```python
from build123d import *

# Parameters (mm, degrees)
SKETCH1_W           = 155.575
SKETCH1_H           = 107.237500028
BOSS_EXTRUDE1_DEPTH = 36.5
SHELL2_T            = -3.175
FILLET1_R           = 2.54
CUT_EXTRUDE2_REACH  = 194.447
SKETCH7_R           = 1.2
SKETCH7_W           = 15
SKETCH7_H           = 15
SKETCH8_R           = 2.38125
CUT_EXTRUDE3_DEPTH  = 190.889155594


with BuildPart() as part:
    # Sketch1 → Boss-Extrude1 (new body)
    with BuildSketch(Plane(origin=(0, 0, 0), x_dir=(0, 0, -1), z_dir=(1, 0, 0))):
        with Locations((77.7875, 53.618750014)):
            Rectangle(SKETCH1_W, SKETCH1_H)
    extrude(amount=BOSS_EXTRUDE1_DEPTH)

    # Shell2
    shell2_openings = [part.faces().sort_by_distance(p)[0] for p in [
        (18.25, 53.618750014, 0),
    ]]
    offset(amount=SHELL2_T, openings=shell2_openings, kind=Kind.INTERSECTION)

    # Fillet1
    fillet1_edges = [part.edges().sort_by_distance(p)[0] for p in [
        (36.5, 107.237500028, -77.7875),
        (0, 107.237500028, -77.7875),
        (0, 0, -77.7875),
        (36.5, 0, -77.7875),
    ]]
    fillet(fillet1_edges, radius=FILLET1_R)

    # Sketch7 → Cut-Extrude2 (cut, up to next)
    with BuildSketch(Plane(origin=(0, 0, -155.575), x_dir=(-1, 0, 0), z_dir=(0, 0, -1)), mode=Mode.PRIVATE) as cut_extrude2_sk1:
        with Locations((-7.175, 30)):
            Circle(SKETCH7_R)
    cut_extrude2_tool1 = extrude(cut_extrude2_sk1.sketch, amount=-CUT_EXTRUDE2_REACH, mode=Mode.PRIVATE) & part.part
    # Sketch7 → Cut-Extrude2 (cut, up to next)
    with BuildSketch(Plane(origin=(0, 0, -155.575), x_dir=(-1, 0, 0), z_dir=(0, 0, -1)), mode=Mode.PRIVATE) as cut_extrude2_sk2:
        with Locations((-7.175, 5)):
            Circle(SKETCH7_R)
    cut_extrude2_tool2 = extrude(cut_extrude2_sk2.sketch, amount=-CUT_EXTRUDE2_REACH, mode=Mode.PRIVATE) & part.part
    # Sketch7 → Cut-Extrude2 (cut, up to next)
    with BuildSketch(Plane(origin=(0, 0, -155.575), x_dir=(-1, 0, 0), z_dir=(0, 0, -1)), mode=Mode.PRIVATE) as cut_extrude2_sk3:
        with Locations((-20.675, 27.5)):
            Rectangle(SKETCH7_W, SKETCH7_H)
    cut_extrude2_tool3 = extrude(cut_extrude2_sk3.sketch, amount=-CUT_EXTRUDE2_REACH, mode=Mode.PRIVATE) & part.part
    add(cut_extrude2_tool1.solids().sort_by_distance((7.175, 30, -155.575))[0], mode=Mode.SUBTRACT)
    add(cut_extrude2_tool2.solids().sort_by_distance((7.175, 5, -155.575))[0], mode=Mode.SUBTRACT)
    add(cut_extrude2_tool3.solids().sort_by_distance((20.675, 27.5, -155.575))[0], mode=Mode.SUBTRACT)

    # Sketch8 → Cut-Extrude3 (cut, through all)
    with BuildSketch(Plane.XY.offset(-152.4)):
        with Locations((7.175, 25.4)):
            Circle(SKETCH8_R)
    extrude(amount=-CUT_EXTRUDE3_DEPTH, mode=Mode.SUBTRACT)


solid = part.part
```
Geometry: final body of the model. Coordinates: model frame, mm. A direction names the side the tool comes from. Coordinates: 2 decimals unless noted, no trailing zeros. Order: outer loops, then holes, each group sorted by start corner. A loop starts at its lowest first (then second) coordinate and runs counter-clockwise, first axis right, second up.
Item 1: Section query A-A (x = 23.5). Output: boundary loops of the cut face in (y, z) (1 decimal).
Answer:
outline: (0, -155.6) - (20, -155.6) - (20, -152.4) - (3.2, -152.4) - (3.2, 0) - (0, 0) - close; (35, -155.6) - (107.2, -155.6) - (107.2, 0) - (104.1, 0) - (104.1, -152.4) - (35, -152.4) - close
Item 2: Draft query along X for faces 4 (the face through (28.175, 27, -154)), 5 (the face through (18, 107.238, -77)), 6 (the face through (36.5, 54, -77)), 7 (the face through (18, 53, -152.4)). Return one class per face: released by +X, released by -X, zero draft, split by the parting line, or undercut.
Answer:
face 4: undercut
face 5: zero draft
face 6: released by +X
face 7: undercut
Item 3: Material intervals for line 1 along Y through (x, z) = (28, -130) (1 decimal); line 2 along X through (y, z) = (51, -79.5) (3 decimals); line 3 along Z through (x, y) = (16.5, 12.5) (3 decimals), sorted ascending.
Answer:
line 1: y = 0 to 3.2, 104.1 to 107.2
line 2: x = 0 to 3.175, 33.325 to 36.5
line 3: z = -155.575 to -152.4
Item 4: Contact query for a flat-ended pin moving along its axis: P1, Ø4, axis at x = 8.5, y = 41, coming from the +Z side. Output: stop coordinate, or through.
Answer:
P1: stops at z = -152.4
Item 5: Section query D-D (y = 25.4). Output: boundary loops of the cut face in (x, z) (3 decimals).
Answer:
outline: (0, -155.575) - (4.794, -155.575) - (4.794, -152.4) - (3.175, -152.4) - (3.175, 0) - (0, 0) - close; (9.556, -155.575) - (13.175, -155.575) - (13.175, -152.4) - (9.556, -152.4) - close; (28.175, -155.575) - (36.5, -155.575) - (36.5, 0) - (33.325, 0) - (33.325, -152.4) - (28.175, -152.4) - close
Item 6: Section query B-B (z = -138). Output: boundary loops of the cut face in (x, y) (1 decimal).
Answer:
outline: (0, 2.5) arc R2.5 ccw to (2.5, 0) - (34, 0) arc R2.5 ccw to (36.5, 2.5) - (36.5, 104.7) arc R2.5 ccw to (34, 107.2) - (2.5, 107.2) arc R2.5 ccw to (0, 104.7) - close; hole (3.2, 3.2) - (33.3, 3.2) - (33.3, 104.1) - (3.2, 104.1) - close
Item 7: Section query C-C (y = 61). Output: boundary loops of the cut face in (x, z) (3 decimals).
Answer:
outline: (0, -155.575) - (36.5, -155.575) - (36.5, 0) - (33.325, 0) - (33.325, -152.4) - (3.175, -152.4) - (3.175, 0) - (0, 0) - close
Item 8: Access query for faces 1 (the face through (18, 3.175, -75)), 2 (the face through (21, 35, -154)), 3 (the face through (34, 49, 0)). Directions: +Z, -Z, +X, -X, +Y, -Y. A direction counts if a zero-diameter tool reaches every point of the face in a straight line with its end or side. Return the directions, or none.
Answer:
face 1: +Z
face 2: +Z, -Z
face 3: +Z, +X, -X, +Y, -Y
